```python
from build123d import *

# Parameters (mm, degrees)
SKETCH1_R           = 3.25
SKETCH1_R_2         = 2.38125
BOSS_EXTRUDE1_DEPTH = 4


with BuildPart() as part:
    # Sketch1 → Boss-Extrude1 (new body)
    with BuildSketch(Plane(origin=(0, 0, 0), x_dir=(1, 0, 0), z_dir=(0, 1, 0))):
        with BuildLine():
            Line((-50.8, 12.7), (50.8, 12.7))
            ThreePointArc((50.8, 12.7), (63.5, 0), (50.8, -12.7))
            Line((50.8, -12.7), (-50.8, -12.7))
            ThreePointArc((-50.8, -12.7), (-63.5, 0), (-50.8, 12.7))
        make_face()
        with Locations(Location((-50.8, 0, 0), (0, 0, 270))):
            Circle(SKETCH1_R, mode=Mode.SUBTRACT)
        with Locations(Location((50.8, 0, 0), (0, 0, 270))):
            Circle(SKETCH1_R_2, mode=Mode.SUBTRACT)
        with BuildLine():
            Line((-56.81040764, 7.778174593), (-54.689087297, 5.656854249))
            ThreePointArc((-54.689087297, 5.656854249), (-54.689087297, 3.889087297), (-56.456854249, 3.889087297))
            Line((-56.456854249, 3.889087297), (-58.578174593, 6.01040764))
            ThreePointArc((-58.578174593, 6.01040764), (-58.578174593, 7.778174593), (-56.81040764, 7.778174593))
        make_face(mode=Mode.SUBTRACT)
        with BuildLine():
            Line((-43.021825407, 6.01040764), (-45.143145751, 3.889087297))
            ThreePointArc((-45.143145751, 3.889087297), (-46.910912703, 3.889087297), (-46.910912703, 5.656854249))
            Line((-46.910912703, 5.656854249), (-44.78959236, 7.778174593))
            ThreePointArc((-44.78959236, 7.778174593), (-43.021825407, 7.778174593), (-43.021825407, 6.01040764))
        make_face(mode=Mode.SUBTRACT)
        with BuildLine():
            Line((-44.78959236, -7.778174593), (-46.910912703, -5.656854249))
            ThreePointArc((-46.910912703, -5.656854249), (-46.910912703, -3.889087297), (-45.143145751, -3.889087297))
            Line((-45.143145751, -3.889087297), (-43.021825407, -6.01040764))
            ThreePointArc((-43.021825407, -6.01040764), (-43.021825407, -7.778174593), (-44.78959236, -7.778174593))
        make_face(mode=Mode.SUBTRACT)
        with BuildLine():
            Line((-58.578174593, -6.01040764), (-56.456854249, -3.889087297))
            ThreePointArc((-56.456854249, -3.889087297), (-54.689087297, -3.889087297), (-54.689087297, -5.656854249))
            Line((-54.689087297, -5.656854249), (-56.81040764, -7.778174593))
            ThreePointArc((-56.81040764, -7.778174593), (-58.578174593, -7.778174593), (-58.578174593, -6.01040764))
        make_face(mode=Mode.SUBTRACT)
    extrude(amount=BOSS_EXTRUDE1_DEPTH)


solid = part.part
```
Here's how the part is built. I have some questions about the finished solid (model axes, mm). A direction names the side the tool comes from. Coordinates: 2 decimals unless noted, no trailing zeros. Write each loop counter-clockwise with the first axis right and the second up, starting at its lowest first coordinate (ties: lowest second). Pieces come first, ordered by that corner, then holes. Notation, with made-up numbers: (-9.5, 29) - (28.5, 29) arc R27 cw to (28.5, 46) - close; hole circle Ø3 at (37, -21). An arc over 180 degrees is marked (long way). One line per item, written item: value.
1) I'm going to push flat-ended pins straight in: P1, Ø5, axis at x = -50.8, z = 0, coming from the -Y side; P2, Ø1.5, axis at y = 2, z = -1.5, coming from the -X side. Where does each tip first touch, or does it pass through?
Model answer:
P1: passes through
P2: stops at x = -63.48
2) Suppose I cut it at A-A on y = 2.6. Write out the boundary of the cut face in (x, z), and give its area (3 significant figures).
Model answer:
outline: (-50.8, -12.7) - (50.8, -12.7) arc R12.7 ccw to (50.8, 12.7) - (-50.8, 12.7) arc R12.7 ccw to start; hole (-58.58, -6.01) arc R1.25 ccw to (-56.81, -7.78) - (-54.69, -5.66) arc R1.25 ccw to (-56.46, -3.89) - close; hole (-58.58, 6.01) - (-56.46, 3.89) arc R1.25 ccw to (-54.69, 5.66) - (-56.81, 7.78) arc R1.25 ccw to start; hole circle Ø6.5 at (-50.8, 0); hole (-46.91, -5.66) - (-44.79, -7.78) arc R1.25 ccw to (-43.02, -6.01) - (-45.14, -3.89) arc R1.25 ccw to start; hole (-46.91, 5.66) arc R1.25 ccw to (-45.14, 3.89) - (-43.02, 6.01) arc R1.25 ccw to (-44.79, 7.78) - close; hole circle Ø4.76 at (50.8, 0)
area: 2,990 mm²
3) I need wall thicknesses on line 1 along X through (y, z) = (2.6, 0); line 2 along X through (y, z) = (1.2, -7.5); line 3 along X through (y, z) = (1.95, 2.75). Which ranges of each line are inside material? Lowest first, please.
Model answer:
line 1: x = -63.5 to -54.05, -47.55 to 48.42, 53.18 to 63.5
line 2: x = -61.05 to -58.79, -56.53 to -45.07, -42.81 to 61.05
line 3: x = -63.2 to -52.53, -49.07 to 63.2
4) We'd pull the mould along Z, two halves only. Please class faces 1 (the flat face through (-45.84, 1.97, 6.73)), 2 (the cylindrical face through (63.497, 1.972, -0.279)), 3 (the flat face through (1, 4, 0)), 4 (the flat face through (-57.5, 1.97, -4.93)): pulls with the +Z half, pulls with the -Z half, needs draft (parallel to the pull), parting line crosses it, or undercut.
Model answer:
face 1: undercut
face 2: parting line crosses it
face 3: needs draft
face 4: undercut
5) Suppose I cut it at C-C on z = -9.75. Write out the boundary of the cut face in (x, y), and give its area (3 significant figures).
Model answer:
outline: (-58.94, 0) - (58.94, 0) - (58.94, 4) - (-58.94, 4) - close
area: 472 mm²
6) On a 3-axis mill with a long thin cutter (end or side, diameter ignored), from which of +Z, -Z, +X, -X, +Y, -Y can I reach the whole of each face in a straight line? I mean faces 5 (the flat face through (-55.73, 1.97, 6.7)), 6 (the flat face through (1, 2, 12.7)). Say none if no direction works.
Model answer:
face 5: +Y, -Y
face 6: +Z, +X, -X, +Y, -Y
7) Suppose I cut it at B-B on z = 0. Write out the boundary of the cut face in (x, y).
Model answer:
outline: (-63.5, 0) - (-54.05, 0) - (-54.05, 4) - (-63.5, 4) - close; (-47.55, 0) - (48.42, 0) - (48.42, 4) - (-47.55, 4) - close; (53.18, 0) - (63.5, 0) - (63.5, 4) - (53.18, 4) - close
